Autodesk Inventor part; units mm, degrees
ref_plane "YZ Plane" through (0, 0, 0) normal (1, 0, 0) x (0, 1, 0)
ref_plane "XZ Plane" through (0, 0, 0) normal (0, 1, 0) x (-1, 0, 0)
ref_plane "XY Plane" through (0, 0, 0) normal (0, 0, 1) x (1, 0, 0)
sketch "Boceto1" plane through (0, 0, 0) normal (0, 1, 0) x (-1, 0, 0)
  line L0 (9.0866, 25.3081) -> (-54.4134, 25.3081)
  line L1 (-54.4134, 25.3081) -> (-54.4134, 8.8081)
  line L2 (-54.4134, 8.8081) -> (9.0866, 8.8081)
  line L3 (9.0866, 8.8081) -> (9.0866, 25.3081)
  arc A0 (-0.7134, 17.3081) -> (4.2866, 17.3081) centre (1.7866, 17.3081) ccw
  arc A1 (-25.1634, 18.3081) -> (-20.1634, 18.3081) centre (-22.6634, 18.3081) ccw
  arc A2 (-48.6134, 17.3081) -> (-43.6134, 17.3081) centre (-46.1134, 17.3081) ccw
  line L4 (4.2866, 17.3081) -> (4.2866, 21.3081)
  line L5 (-0.7134, 17.3081) -> (-0.7134, 21.3081)
  arc A3 (4.2866, 21.3081) -> (-0.7134, 21.3081) centre (1.7866, 21.3081) ccw
  line L6 (-43.6134, 17.3081) -> (-43.6134, 21.3081)
  line L7 (-48.6134, 17.3081) -> (-48.6134, 21.3081)
  arc A4 (-43.6134, 21.3081) -> (-48.6134, 21.3081) centre (-46.1134, 21.3081) ccw
  line L8 (-20.1634, 18.3081) -> (-20.1634, 21.8081)
  line L9 (-25.1634, 18.3081) -> (-25.1634, 21.8081)
  arc A5 (-20.1634, 21.8081) -> (-25.1634, 21.8081) centre (-22.6634, 21.8081) ccw
  point P0 (0, 0)
  dimension "d1" = 16.5
  dimension "d2" = 5
  dimension "d3" = 5
  dimension "d4" = 5
  dimension "d10" = 7
  dimension "d11" = 31.75
  dimension "d12" = 8
  dimension "d13" = 8.3
  dimension "d14" = 63.5
  dimension "d15" = 8
  dimension "d16" = 7.3
  dimension "d30" = 4
  dimension "d31" = 4
  dimension "d32" = 4
  dimension "d33" = 4
  dimension "d34" = 3.5
  dimension "d35" = 3.5
extrude "Extrusión1" add sketch "Boceto1" along normal blind 1.2
sketch "Boceto2" plane through (54.4134, 0, 25.3081) normal (1, 0, 0) x (0, 0, -1)
  circle A0 centre (18.875, 2.375) radius 2.375
  circle A1 centre (18.875, 2.375) radius 1.625
  line L0 (16.5, 0) -> (16.5, 1.2)
  line L1 (0, 0) -> (16.5, 0)
  line L2 (16.5, 0) -> (16.5, 1.2)
  line L3 (16.5, 1.2) -> (16.5, 2.375)
  line L4 (16.5, 1.2) -> (16.5, 0)
  line L5 (16.5, 0) -> (18.875, 0)
  point P0 (25.3081, 0)
  dimension "d19" = 4.75
  dimension "d20" = 3.25
extrude "Extrusión2" add sketch "Boceto2" against normal blind 63.5
sketch "Boceto3" plane through (0, 0, 0) normal (0, -1, 0) x (1, 0, 0)
  line L0 (54.4134, 8.8081) -> (-9.0866, 8.8081)
  line L1 (-9.0866, 8.8081) -> (54.4134, 8.8081)
  line L2 (22.6634, 8.8081) -> (35.6634, 8.8081)
  line L3 (35.6634, 8.8081) -> (9.6634, 8.8081)
  line L4 (9.6634, 8.8081) -> (9.6634, -4.6873)
  line L5 (9.6634, -4.6873) -> (35.6634, -4.6873)
  line L6 (35.6634, -4.6873) -> (35.6634, 8.8081)
  point P0 (0, 0)
  dimension "d23" = 13
  dimension "d24" = 26
extrude "Extrusión3" cut sketch "Boceto3" against normal blind 63.5
chamfer "Chaflán1" distance 0.25 angle 45 3 edges at (22.6634, 1.2, 15.8081) (-1.7866, 1.2, 14.8081) (46.1134, 1.2, 14.8081)
properties part number "Ala 1 Bisagra tipo T"
Verification items for the finished model (mm, model axes). A direction names the side the tool comes from. Round coordinates to 2 decimals unless told otherwise and drop trailing zeros. Order: outer loops, then holes, each group sorted by start corner. A loop starts at its lowest first (then second) coordinate and runs counter-clockwise, first axis right, second up. Notation, with made-up numbers: (45, 21) -> (70, 21) arc R14 cw to (70, 29) -> close; hole circle Ø1 at (11, 16). An arc over 180 degrees is marked (long way). Put each result on its own line as item: value. Start each with the question number.
(1) Material ranges on line 1 along X through (y, z) = (0.3, 7.25); line 2 along Y through (x, z) = (-1, 12); line 3 along Y through (x, z) = (51, 7), recorded low to high.
(2) Draft check along Z on faces 5 (the face through (46.17, 1.08, 14.68)), 6 (the face through (35.663, 1, 8)), 7 (the face through (0, 2, 8.808)), 8 (the face through (45.17, 2.446, 8.057)). Enter one of: +Z half, -Z half, draft (parallel to the pull), parting line (faces both ways), or undercut.
(3) Tool access check on faces 1 (the face through (-1.732, 0.468, 23.807)), 2 (the face through (23, 1.2, 15)), 3 (the face through (45.2, 4, 4.7)), 4 (the face through (22.606, 1.077, 24.434)). Record the directions out of +Z, -Z, +X, -X, +Y, -Y that give a thin tool (end or side, any length) a straight path to the whole face; none if there is none.
(4) Section check D-D (z = 7.25). Enter the section's corners in (x, y), then the cut area to 3 significant figures.
(5) Section check C-C (x = 42). Enter the section's corners in (y, z) (3 decimals).
(6) Section check B-B (y = 1.8). Enter the section's corners in (x, z), then the cut area to 3 significant figures.
(7) Section check A-A (z = 20.25). Enter the section's corners in (x, y).
(8) Depth check by flat-ended pin: pin 1 Ø8 at (x, z) = (21, 22) entering from +Y; pin 2 Ø0.6 at (x, y) = (49.5, 2) entering from +Z. Enter the tip coordinate at first touch or a pass-through.
Completed:
1. line 1: x = -9.09 to 9.66, 35.66 to 54.41
1. line 2: y = 0 to 1.2
1. line 3: y = 0 to 0.85, 3.9 to 4.68
2. face 5: undercut
2. face 6: draft
2. face 7: +Z half
2. face 8: undercut
3. face 1: +Y, -Y
3. face 2: +Z, +X, -X, +Y
3. face 3: +X, -X
3. face 4: +Y
4. outline: (-9.09, 0) -> (9.66, 0) -> (9.66, 0.97) -> (-9.09, 0.97) -> close; (-9.09, 3.78) -> (9.66, 3.78) -> (9.66, 4.61) -> (-9.09, 4.61) -> close; (35.66, 0) -> (54.41, 0) -> (54.41, 0.97) -> (35.66, 0.97) -> close; (35.66, 3.78) -> (54.41, 3.78) -> (54.41, 4.61) -> (35.66, 4.61) -> close
4. area: 67.3 mm2
5. outline: (0, 6.433) arc R2.375 ccw (long way) to (2.375, 8.808) -> (1.2, 8.808) -> (1.2, 25.308) -> (0, 25.308) -> close; hole circle Ø3.25 at (2.375, 6.433)
6. outline: (-9.09, 4.13) -> (9.66, 4.13) -> (9.66, 4.91) -> (-9.09, 4.91) -> close; (-9.09, 7.95) -> (9.66, 7.95) -> (9.66, 8.81) -> (-9.09, 8.81) -> close; (35.66, 4.13) -> (54.41, 4.13) -> (54.41, 4.91) -> (35.66, 4.91) -> close; (35.66, 7.95) -> (54.41, 7.95) -> (54.41, 8.81) -> (35.66, 8.81) -> close
6. area: 61.5 mm2
7. outline: (-9.09, 0) -> (-4.29, 0) -> (-4.29, 0.95) -> (-4.54, 1.2) -> (-9.09, 1.2) -> close; (0.71, 0) -> (20.16, 0) -> (20.16, 0.95) -> (19.91, 1.2) -> (0.96, 1.2) -> (0.71, 0.95) -> close; (25.16, 0) -> (43.61, 0) -> (43.61, 0.95) -> (43.36, 1.2) -> (25.41, 1.2) -> (25.16, 0.95) -> close; (48.61, 0) -> (54.41, 0) -> (54.41, 1.2) -> (48.86, 1.2) -> (48.61, 0.95) -> close
8. pin 1: stops at y = 1.2
8. pin 2: stops at z = 8.81
